```python
from build123d import *

# Parameters (mm, degrees)
F1_DEPTH = 20
F2_R     = 2
F3_DEPTH = 19.001
F4_R     = 2
F5_DEPTH = 8
F6_SIZE  = 1


with BuildPart() as f1:
    # F0 (on Top) → F1 (new body)
    with BuildSketch(Plane.XY):
        with BuildLine():
            Line((-9, 9.5), (-19, 9.5))
            Line((-19, 9.5), (-19, -9.5))
            Line((-19, -9.5), (19, -9.5))
            Line((19, -9.5), (19, 9.5))
            Line((19, 9.5), (9, 9.5))
            ThreePointArc((9, 9.5), (0, 0.5), (-9, 9.5))
        make_face()
    extrude(amount=F1_DEPTH)

    # F2 (on face) → F3 (cut, through all)
    with BuildSketch(Plane(origin=(0, 9.5, 0), x_dir=(-1, 0, 0), z_dir=(0, 1, 0))):
        with Locations((-14, 10)):
            Circle(F2_R)
        with Locations((14, 10)):
            Circle(F2_R)
    extrude(amount=-F3_DEPTH, mode=Mode.SUBTRACT)

    # F4 (on face) → F5 (cut)
    with BuildSketch(Plane.XZ.offset(9.5)):
        with Locations((0, 10)):
            Circle(F4_R)
    extrude(amount=-F5_DEPTH, mode=Mode.SUBTRACT)

    # F6
    f6_edges = [f1.edges().sort_by_distance(p)[0] for p in [
        (0, 0.5, 0),
        (0, 0.5, 20),
    ]]
    chamfer(f6_edges, length=F6_SIZE)


solid = f1.part
```
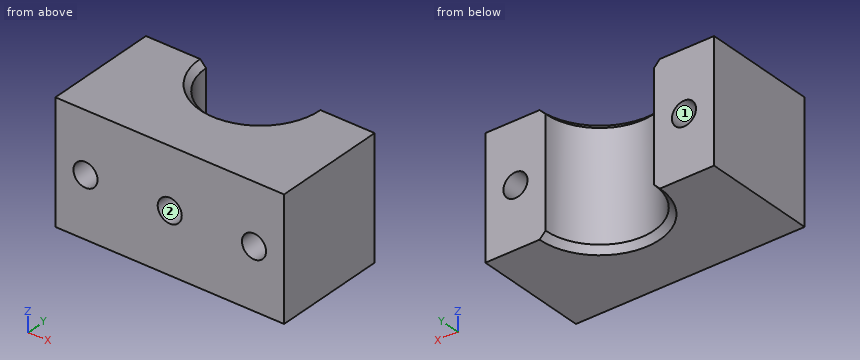
For this review, take the finished solid that the model builds, in its own axes (mm). Face numbers are marked on the shaded views. A direction names the side the tool comes from. Round coordinates to 2 decimals unless told otherwise and drop trailing zeros. Write each loop counter-clockwise with the first axis right and the second up, starting at its lowest first coordinate (ties: lowest second). Pieces come first, ordered by that corner, then holes. Notation, with made-up numbers: M 81,63.5 L 124,63.5 A22 ccw 124,69.5 Z; hole C 10.5,8.5 d4. An arc over 180 degrees is marked long. One line per item, written item: value. Start each with the question number.
(1) We need section C-C (z = 10). Give the boundary of the cut face in (x, y), and give its area (3 significant figures).
(2) Wall thickness on line 1 (Z direction, x = -14, y = -2.25); line 2 (X direction, y = 6.75, z = 11.25); line 3 (X direction, y = 2, z = 10.75): over which ranges is each line inside the solid? List them lowest first.
(3) We need section B-B (y = -3.5). Give the boundary of the cut face in (x, z), and give its area (3 significant figures).
(4) We need section A-A (x = -14). Give the boundary of the cut face in (y, z), and give its area (3 significant figures).
(5) Machinability: for the marked faces 1 and 2, which of the approach directions +Z, -Z, +X, -X, +Y, -Y give a long, thin tool a straight path to every point of the face, cutting with its end or side? Answer none if there is none.
(6) We need section D-D (z = 2). Give the boundary of the cut face in (x, y), and give its area (3 significant figures).
Result:
1. outline: M -19,-9.5 L -16,-9.5 L -16,9.5 L -19,9.5 Z; M -12,-9.5 L -2,-9.5 L -2,-1.5 L 2,-1.5 L 2,-9.5 L 12,-9.5 L 12,9.5 L 9,9.5 A9 cw -9,9.5 L -12,9.5 Z; M 16,-9.5 L 19,-9.5 L 19,9.5 L 16,9.5 Z
1. area: 411 mm²
2. line 1: 0 to 8, 12 to 20
2. line 2: -19 to -15.56, -12.44 to -8.57, 8.57 to 12.44, 15.56 to 19
2. line 3: -19 to -15.85, -12.15 to -4.97, 4.97 to 12.15, 15.85 to 19
3. outline: M -19,0 L 19,0 L 19,20 L -19,20 Z; hole C -14,10 d4; hole C 0,10 d4; hole C 14,10 d4
3. area: 722 mm²
4. outline: M -9.5,0 L 9.5,0 L 9.5,8 L -9.5,8 Z; M -9.5,12 L 9.5,12 L 9.5,20 L -9.5,20 Z
4. area: 304 mm²
5. face 1: +Y, -Y
5. face 2: -Y
6. outline: M -19,-9.5 L 19,-9.5 L 19,9.5 L 9,9.5 A9 cw -9,9.5 L -19,9.5 Z
6. area: 595 mm²
